```python
from build123d import *

# Parameters (mm, degrees)
PAD_DEPTH    = 35
PAD001_DEPTH = 20
POCKET_DEPTH = 100.001


with BuildPart() as part:
    # Sketch → Pad (new body, symmetric)
    with BuildSketch(Plane.XZ):
        Polygon((0, 100), (0, 0), (75, 0), (75, 20), (25, 20), (25, 80), align=None)
    extrude(amount=PAD_DEPTH, both=True)

    # Sketch001 → Pad001 (join)
    with BuildSketch(Plane.XY):
        with BuildLine():
            ThreePointArc((75, -35), (110, 0), (75, 35))
            Line((75, 35), (75, -35))
        make_face()
    extrude(amount=PAD001_DEPTH)

    # Sketch002 → Pocket (cut, through all)
    with BuildSketch(Plane.XY):
        Polygon((0, 10), (0, -10), (12, -16.928203), (12, 16.928203), align=None)
        Polygon((57.679492, -10), (75, -20), (92.320508, -10), (92.320508, 10), (75, 20), (57.679492, 10), align=None)
    extrude(amount=POCKET_DEPTH, mode=Mode.SUBTRACT)


solid = part.part
```
Geometry: final body of the model. Coordinates: model frame, mm. A direction names the side the tool comes from. Give positions to 0.01 mm unless a question says otherwise; leave off trailing zeros. Write each loop counter-clockwise with the first axis right and the second up, starting at its lowest first coordinate (ties: lowest second). Pieces come first, ordered by that corner, then holes.
1. Line query: probe 1 along X at (y, z) = (7.5, 21); probe 2 along X at (y, z) = (17, 72.5); probe 3 along Z at (x, y) = (41, 12.5). Output: solid intervals per line, ascending.
2. Pin query (flat end, axial travel): P1, Ø1, axis at y = -23, z = 17, coming from the +X side; P2, Ø6, axis at x = 73.5, y = 26.5, coming from the +Z side; P3, Ø6, axis at y = 23, z = 89, coming from the -X side; P4, Ø22, axis at y = 3.5, z = 5, coming from the +X side. Return the tip coordinate at first contact, or that it passes through.
3. Section query B-B, the plane x = 76.5. Return loops of the section in (y, z), then the cut area to 3 significant figures.
4. Reachability of faces 1 (the flat face through (20, -35, 40)), 2 (the flat face through (5.92, -13.42, 49.3)), 3 (the flat face through (57, 0, 20)) from +Z, -Z, +X, -X, +Y, -Y: full face, straight path, thin tool, end or side. Return the list, or none.
5. Section query D-D, the plane y = 14. Return loops of the section in (x, z), then the cut area to 3 significant figures.
6. Draft query along X for faces 4 (the flat face through (20, 35, 40)), 5 (the flat face through (0, 22, 51)), 6 (the flat face through (83.78, 14.93, 9.86)), 7 (the flat face through (25, 0, 50)). Return one class per face: released by +X, released by -X, zero draft, split by the parting line, or undercut.
7. Section query C-C, the plane z = 27. Return loops of the section in (x, y).
8. Section query A-A, the plane y = 0. Return loops of the section in (x, z), then the cut area to 3 significant figures.
Computed:
1. probe 1: x = 12 to 25
1. probe 2: x = 0 to 25
1. probe 3: z = 0 to 20
2. P1: stops at x = 101.81
2. P2: stops at z = 20
2. P3: stops at x = 0
2. P4: stops at x = 110
3. outline: (-34.97, 0) - (-19.13, 0) - (-19.13, 20) - (-34.97, 20) - close; (19.13, 0) - (34.97, 0) - (34.97, 20) - (19.13, 20) - close
3. area: 633 mm2
4. face 1: +Z, -Z, +X, -X, -Y
4. face 2: +Z, -Z
4. face 3: +Z, +X, +Y, -Y
5. outline: (0, 0) - (6.93, 0) - (6.93, 94.46) - (0, 100) - close; (12, 0) - (64.61, 0) - (64.61, 20) - (25, 20) - (25, 80) - (12, 90.4) - close; (85.39, 0) - (107.08, 0) - (107.08, 20) - (85.39, 20) - close
5. area: 3,010 mm2
6. face 4: zero draft
6. face 5: released by -X
6. face 6: undercut
6. face 7: released by +X
7. outline: (0, -35) - (25, -35) - (25, 35) - (0, 35) - (0, 10) - (12, 16.93) - (12, -16.93) - (0, -10) - close
8. outline: (12, 0) - (57.68, 0) - (57.68, 20) - (25, 20) - (25, 80) - (12, 90.4) - close; (92.32, 0) - (110, 0) - (110, 20) - (92.32, 20) - close
8. area: 2,110 mm2
